```python
from build123d import *

# Parameters (mm, degrees)
F0_W     = 60
F0_H     = 90
F1_DEPTH = 12
F2_D     = 13


with BuildPart() as f1:
    # F0 (on Front) → F1 (new body)
    with BuildSketch(Plane.XZ):
        with Locations((-9.5794885419, 35.4121185594)):
            Rectangle(F0_W, F0_H)
    extrude(amount=F1_DEPTH)

    # F2 (through all)
    with Locations(Plane(origin=(0, 0, 0), x_dir=(1, 0, 0), z_dir=(0, 1, 0))):
        with Locations((-24.5794885419, -62.9121185594), (-24.5794885419, -7.9121185594)):
            Hole(F2_D / 2)


solid = f1.part
```
Verification items for the finished model (mm, model axes). Give positions to 0.01 mm unless a question says otherwise; leave off trailing zeros. Order: outer loops, then holes, each group sorted by start corner. A loop starts at its lowest first (then second) coordinate and runs counter-clockwise, first axis right, second up. Notation, with made-up numbers: (-13, 65) - (35, 65) arc R29 ccw to (35, 101) - close; hole circle Ø8 at (-16, -21.5). An arc over 180 degrees is marked (long way). Answer as CSV lines item,"result". Start each with the question number.
Item 1: Section check B-B, the plane y = -8. Record the boundary of the cut face in (x, z).
Item 2: Mould release check, pull along Z, two halves, no side actions. Record for faces 1 (the face through (20.421, -6, 35)), 2 (the face through (-23.733, -6.084, 56.467)), 3 (the face through (-10, -6, -9.588)): released by +Z, released by -Z, zero draft, split by the parting line, or undercut.
Item 3: Material ranges on L1, parallel to Z at x = -24, y = -0.25; L2, parallel to Z at x = -23, y = -9; L3, parallel to X at y = -8.5, z = 7, recorded low to high.
Item 4: Section check A-A, the plane x = -22. Record the boundary of the cut face in (y, z), plus the area to 3 significant figures.
Filled in:
1,outline,"(-39.58, -9.59) - (20.42, -9.59) - (20.42, 80.41) - (-39.58, 80.41) - close; hole circle Ø13 at (-24.58, 7.91); hole circle Ø13 at (-24.58, 62.91)"
2,face 1,"zero draft"
2,face 2,"undercut"
2,face 3,"released by -Z"
3,L1,"-9.59 to 1.44, 14.39 to 56.44, 69.39 to 80.41"
3,L2,"-9.59 to 1.61, 14.22 to 56.61, 69.22 to 80.41"
3,L3,"-39.58 to -31.02, -18.14 to 20.42"
4,outline,"(-12, -9.59) - (0, -9.59) - (0, 1.95) - (-12, 1.95) - close; (-12, 13.88) - (0, 13.88) - (0, 56.95) - (-12, 56.95) - close; (-12, 68.88) - (0, 68.88) - (0, 80.41) - (-12, 80.41) - close"
4,area,"794 mm^2"
